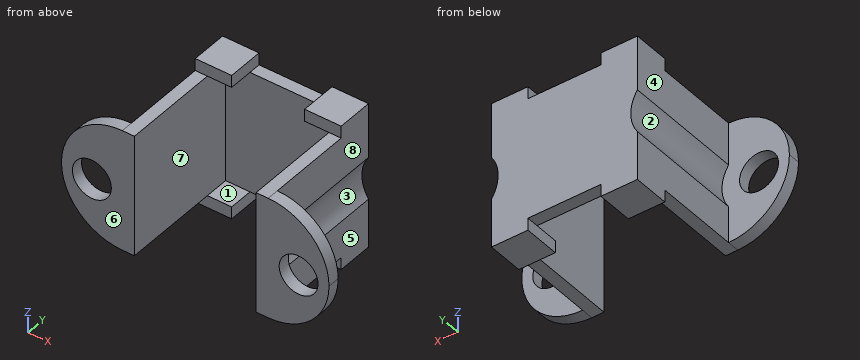
```python
from build123d import *

# Parameters (mm, degrees)
SKETCH1_W           = 6
SKETCH1_H           = 10
BOSS_EXTRUDE1_DEPTH = 1
SKETCH2_W           = 1
SKETCH2_H           = 10
BOSS_EXTRUDE2_DEPTH = 10
SKETCH3_W           = 10
SKETCH3_H           = 1
BOSS_EXTRUDE3_DEPTH = 5
CUT_EXTRUDE1_REACH  = 17.684
SKETCH4_R           = 1.6
CUT_EXTRUDE6_START  = -10
SKETCH5_R           = 3.05
CUT_EXTRUDE6_DEPTH  = 10
SKETCH6_W           = 3
SKETCH6_H           = 3
BOSS_EXTRUDE4_DEPTH = 1
SKETCH7_W           = 3
SKETCH7_H           = 3
BOSS_EXTRUDE5_DEPTH = 1
FILLET2_R           = 5


with BuildPart() as part:
    # Sketch1 → Boss-Extrude1 (new body)
    with BuildSketch(Plane(origin=(0, 0, 0), x_dir=(1, 0, 0), z_dir=(0, 1, 0))):
        with Locations((3, 0)):
            Rectangle(SKETCH1_W, SKETCH1_H)
    extrude(amount=BOSS_EXTRUDE1_DEPTH)

    # Sketch2 → Boss-Extrude2 (add)
    with BuildSketch(Plane.XZ):
        with Locations((5.5, 0)):
            Rectangle(SKETCH2_W, SKETCH2_H)
    extrude(amount=BOSS_EXTRUDE2_DEPTH)

    # Sketch3 → Boss-Extrude3 (add)
    with BuildSketch(Plane(origin=(6, 0, 0), x_dir=(0, 0, -1), z_dir=(1, 0, 0))):
        with Locations((0, -9.5)):
            Rectangle(SKETCH3_W, SKETCH3_H)
    extrude(amount=BOSS_EXTRUDE3_DEPTH)

    # Sketch4 → Cut-Extrude1 (cut, up to next)
    with BuildSketch(Plane(origin=(0, -9, 0), x_dir=(1, 0, 0), z_dir=(0, 1, 0)), mode=Mode.PRIVATE) as cut_extrude1_sk1:
        with Locations(Location((8.5, 0.246614642, 0), (0, 0, 270))):
            Circle(SKETCH4_R)
    cut_extrude1_tool1 = extrude(cut_extrude1_sk1.sketch, amount=-CUT_EXTRUDE1_REACH, mode=Mode.PRIVATE) & part.part
    add(cut_extrude1_tool1.solids().sort_by_distance((8.5, -9, -0.246615))[0], mode=Mode.SUBTRACT)

    # Sketch5 → Cut-Extrude6 (cut)
    with BuildSketch(Plane(origin=(0, 1, 0), x_dir=(1, 0, 0), z_dir=(0, 1, 0)).offset(CUT_EXTRUDE6_START)):
        with Locations((8.5, 0.246614642)):
            Circle(SKETCH5_R)
    extrude(amount=CUT_EXTRUDE6_DEPTH, mode=Mode.SUBTRACT)

    # Sketch6 → Boss-Extrude4 (add)
    with BuildSketch(Plane(origin=(0, 0, -5), x_dir=(-1, 0, 0), z_dir=(0, 0, -1))):
        with Locations((-4.5, -0.5)):
            Rectangle(SKETCH6_W, SKETCH6_H)
    extrude(amount=BOSS_EXTRUDE4_DEPTH)

    # Sketch7 → Boss-Extrude5 (add)
    with BuildSketch(Plane.XY.offset(5)):
        with Locations((4.5, -0.5)):
            Rectangle(SKETCH7_W, SKETCH7_H)
    extrude(amount=BOSS_EXTRUDE5_DEPTH)

    # Fillet2
    fillet2_edges = [part.edges().sort_by_distance(p)[0] for p in [
        (11, -9.5, 5),
        (11, -9.5, -5),
    ]]
    fillet(fillet2_edges, radius=FILLET2_R - 0.0001)  # a hair under: the kernel refuses the full size

    # Mirror1: part across plane


with BuildPart() as part_1:
    add(part.part)
    add(part.part.mirror(Plane(origin=(0, 0, 0), x_dir=(0, 0, 1), z_dir=(1, 0, 0))))


solid = part_1.part
```
Here's how the part is built. I have some questions about the finished solid (model axes, mm). Face numbers are marked on the shaded views. A direction names the side the tool comes from. Round coordinates to 2 decimals unless told otherwise and drop trailing zeros. Write each loop counter-clockwise with the first axis right and the second up, starting at its lowest first coordinate (ties: lowest second). Pieces come first, ordered by that corner, then holes.
Q1. Which directions (+Z, -Z, +X, -X, +Y, -Y) give clear straight access to the entire face, cutting with the end or side of a thin tool? Please do the marked faces 1, 2, 3, 4 and 5.
Q2. If we section it at D-D on x = -8.5: Write out the boundary of the cut face in (y, z).
Q3. If we section it at C-C on z = -0.25: Write out the boundary of the cut face in (x, y).
Q4. Will these pins go through, and if not, where does the flat tip stop? P1, Ø3, axis at y = -5.5, z = 4.5, coming from the -X side; P2, Ø1.5, axis at x = -8, z = -2.5, coming from the +Y side; P3, Ø0.5, axis at x = -1.5, y = 0.5, coming from the -Z side.
Q5. If we section it at B-B on x = -4.75: Write out the boundary of the cut face in (y, z), plus the area to 3 significant figures.
Q6. If we section it at A-A on y = -5: Write out the boundary of the cut face in (x, z), plus the area to 3 significant figures.
Q7. If we mould it in two halves opening along X, with no side actions, what happens to the marked faces 6, 7 and 8? For each: +X half, -X half, draft (parallel to the pull), parting line (faces both ways), or undercut.
Q8. Please list where these lines run through material, in increasing order: probe 1 along X at (y, z) = (-3.5, 4.75); probe 2 along Y at (x, z) = (-8.5, -2); probe 3 along Y at (x, z) = (-4.75, 3.5).
Answer below:
1. face 1: -Y
1. face 2: -X, +Y
1. face 3: +X, +Y
1. face 4: +Z, -Z, -X, +Y
1. face 5: +Z, -Z, +X, +Y
2. outline: (-10, -4.33) - (-9, -4.33) - (-9, -1.85) - (-10, -1.85) - close; (-10, 1.35) - (-9, 1.35) - (-9, 4.33) - (-10, 4.33) - close
3. outline: (-10.99, -10) - (-10.1, -10) - (-10.1, -9) - (-10.99, -9) - close; (-6.9, -10) - (-5, -10) - (-5, 0) - (5, 0) - (5, -10) - (6.9, -10) - (6.9, -9) - (5.45, -9) - (5.45, 1) - (-5.45, 1) - (-5.45, -9) - (-6.9, -9) - close; (10.1, -10) - (10.99, -10) - (10.99, -9) - (10.1, -9) - close
4. P1: stops at x = -6
4. P2: stops at y = -9
4. P3: stops at z = -5
5. outline: (-2, -6) - (1, -6) - (1, 6) - (-2, 6) - (-2, 5) - (0, 5) - (0, -5) - (-2, -5) - close
5. area: 16.0 mm2
6. outline: (-6, -5) - (-5, -5) - (-5, 5) - (-6, 5) - (-6, 1.5) arc R3.05 cw to (-6, -1.99) - close; (5, -5) - (6, -5) - (6, -1.99) arc R3.05 cw to (6, 1.5) - (6, 5) - (5, 5) - close
6. area: 17.4 mm2
7. face 6: draft
7. face 7: undercut
7. face 8: +X half
8. probe 1: x = -6 to -5, 5 to 6
8. probe 2: y = -10 to -9
8. probe 3: y = 0 to 1
